Check sheet for the drawn part. Datum: minimum x, y, z corner. Units: mm. A direction names the side the tool comes from. Round coordinates to 2 decimals unless told otherwise and drop trailing zeros. Write each loop counter-clockwise with the first axis right and the second up, starting at its lowest first coordinate (ties: lowest second). Pieces come first, ordered by that corner, then holes. Notation, with made-up numbers: M 60,8 L 81,8 A15 cw 81,26 Z; hole C 21,14 d7. An arc over 180 degrees is marked long. One line per item, written item: value. Start each with the question number.
1. Depth check by flat-ended pin: P1, Ø2, axis at x = 25, y = 15, coming from the +Z side; P2, Ø8, axis at y = 17, z = 45.5, coming from the +X side; P3, Ø7, axis at x = 47.5, y = 15, coming from the +Z side. Enter the tip coordinate at first touch or a pass-through.
2. Scan lines: probe 1 along X at (y, z) = (33.5, 26.5); probe 2 along Z at (x, y) = (27.5, 11). Record each from-to range of solid material in increasing order. Write a range as [from, to].
3. Release check for a two-part mould opening along X. For the marked faces 3, 4, 5 and 6 record: pulls with the +X half, pulls with the -X half, needs draft (parallel to the pull), parting line crosses it, or undercut.
4. Access from +Z, -Z, +X, -X, +Y, -Y to the whole of each face (thin tool, end or side, straight path). Record for the marked faces 1 and 2.
5. Section check C-C (x = 48). Record the boundary of the cut face in (y, z).
6. Section check D-D (z = 43.5). Record the boundary of the cut face in (x, y).
7. Section check A-A (z = 10). Record the boundary of the cut face in (x, y).
8. Section check B-B (y = 39). Record the boundary of the cut face in (x, z), and give its area (3 significant figures).
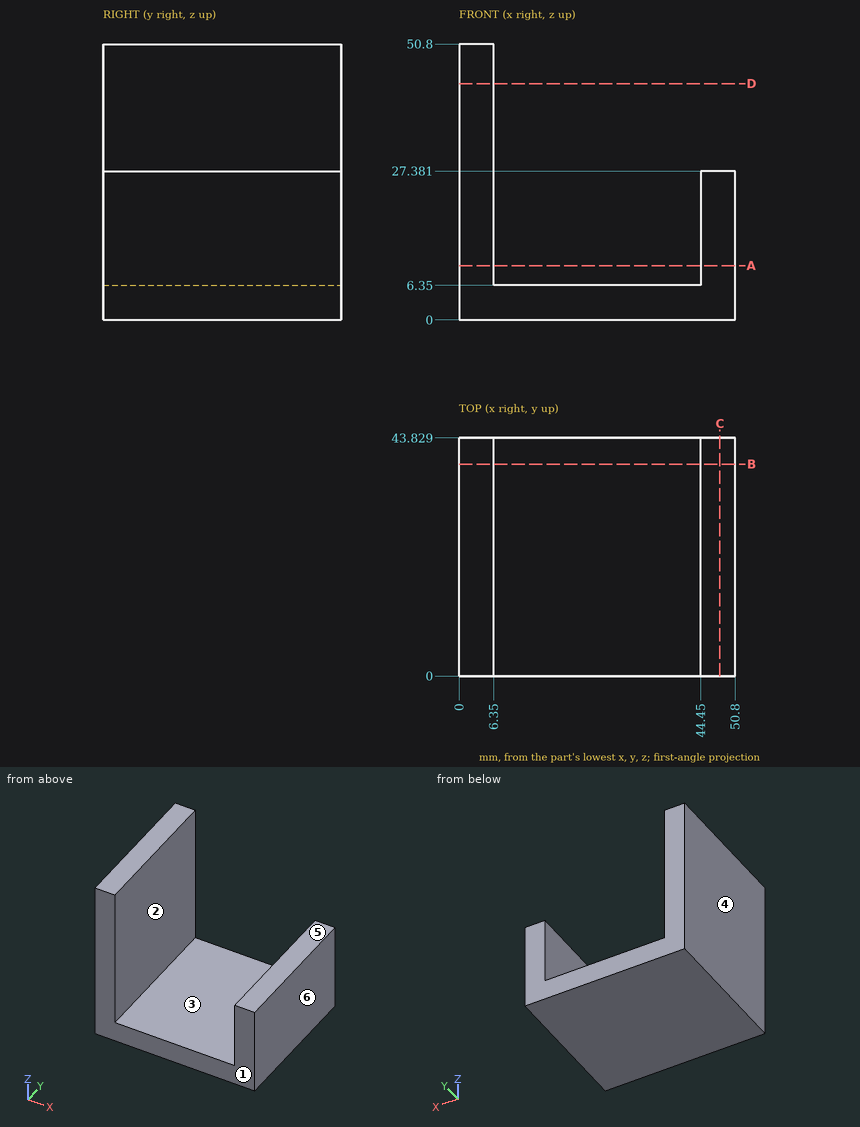
Result sheet:
1. P1: stops at z = 6.35
1. P2: stops at x = 6.35
1. P3: stops at z = 27.38
2. probe 1: x = [0, 6.35], [44.45, 50.8]
2. probe 2: z = [0, 6.35]
3. face 3: undercut
3. face 4: pulls with the -X half
3. face 5: needs draft
3. face 6: pulls with the +X half
4. face 1: +Z, -Z, +X, -X, -Y
4. face 2: +Z, +Y, -Y
5. outline: M 0,0 L 43.83,0 L 43.83,27.38 L 0,27.38 Z
6. outline: M 0,0 L 6.35,0 L 6.35,43.83 L 0,43.83 Z
7. outline: M 0,0 L 6.35,0 L 6.35,43.83 L 0,43.83 Z; M 44.45,0 L 50.8,0 L 50.8,43.83 L 44.45,43.83 Z
8. outline: M 0,0 L 50.8,0 L 50.8,27.38 L 44.45,27.38 L 44.45,6.35 L 6.35,6.35 L 6.35,50.8 L 0,50.8 Z
8. area: 738 mm2
